```python
from build123d import *

# Parameters (mm, degrees)
SKETCH1_R           = 44.45
BOSS_EXTRUDE1_DEPTH = 55.88
SKETCH2_R           = 38.1
CUT_EXTRUDE1_DEPTH  = 22.098
CUT_EXTRUDE2_START  = -28.575
SKETCH3_R           = 38.1
CUT_EXTRUDE2_DEPTH  = 28.575
SKETCH4_R           = 1.27
CUT_EXTRUDE3_DEPTH  = 72.364056247
CUT_EXTRUDE4_DEPTH  = 5


with BuildPart() as part:
    # Sketch1 → Boss-Extrude1 (new body)
    with BuildSketch(Plane.XY):
        Circle(SKETCH1_R)
    extrude(amount=BOSS_EXTRUDE1_DEPTH)

    # Sketch2 → Cut-Extrude1 (cut)
    with BuildSketch(Plane.XY.offset(55.88)):
        Circle(SKETCH2_R)
    extrude(amount=-CUT_EXTRUDE1_DEPTH, mode=Mode.SUBTRACT)

    # Sketch3 → Cut-Extrude2 (cut)
    with BuildSketch(Plane(origin=(0, 0, 0), x_dir=(-1, 0, 0), z_dir=(0, 0, -1)).offset(CUT_EXTRUDE2_START)):
        with Locations(Location((0, 0, 0), (0, 0, 180))):
            Circle(SKETCH3_R)
    extrude(amount=CUT_EXTRUDE2_DEPTH, mode=Mode.SUBTRACT)

    # Sketch4 → Cut-Extrude3 (cut, through all)
    with BuildSketch(Plane.XY.offset(33.782)):
        Circle(SKETCH4_R)
    extrude(amount=-CUT_EXTRUDE3_DEPTH, mode=Mode.SUBTRACT)

    # Sketch5 → Cut-Extrude4 (cut)
    with BuildSketch(Plane.XY.offset(33.782)):
        Polygon((0, 8.082903769), (-7, 4.041451884), (-7, -4.041451884), (0, -8.082903769), (7, -4.041451884), (7, 4.041451884), align=None)
    extrude(amount=-CUT_EXTRUDE4_DEPTH, mode=Mode.SUBTRACT)


solid = part.part
```
Model file for the job. Use its own axes, mm. A direction names the side the tool comes from. Give positions to 0.01 mm unless a question says otherwise; leave off trailing zeros. Loops run counter-clockwise (first coordinate to the right, second up) from the corner with the lowest first, then second, coordinate; pieces in that order, holes last. Notation, with made-up numbers: (17, 16.25) -> (68, 16.25) arc R10 cw to (68, 22.25) -> close; hole circle Ø1 at (25, -17.75). An arc over 180 degrees is marked (long way). Use CSV: the item, a comma, the result in double quotes. Start each with the question number.
1) Mould opens along X. For faces 4 (the flat face through (33, 20, 0)), 5 (the cylindrical face through (42.397, 13.352, 27.549)), 6 (the flat face through (3.549, 6.034, 31.317)) say: released by +X, released by -X, zero draft, split by the parting line, or undercut.
2) Wall check: line 1 (Y direction, x = 0, z = 28); line 2 (Z direction, x = 22.5, y = -13.5) (3 decimals); line 3 (X direction, y = -14, z = 46.5). Give the ranges that are in metal, low to high.
3) Slice it at C-C on x = -23.5. Give the cut face in (y, z) (3 decimals).
4) Flat gauge pins, fed straight in: pin 1 Ø1 at (y, z) = (23.5, 19.5) entering from -X; pin 2 Ø4 at (x, y) = (-2.5, -1) entering from +Z; pin 3 Ø4 at (x, y) = (-15, -28) entering from -Z (3 decimals). Where does each tip first touch, or does it go through?
5) Slice it at B-B on z = 31. Give the cut face in (x, y).
6) Tool access for faces 1 (the flat face through (8, -1, 28.575)), 2 (the flat face through (33, 20, 55.88)), 3 (the flat face through (-3.549, -6.034, 31.317)): list every direction of +Z, -Z, +X, -X, +Y, -Y with a clear straight run to the whole face (end or side of a thin tool).
7) Slice it at D-D on y = -16. Give the cut face in (x, z) (1 decimal), plus the area to 3 significant figures.
8) Slice it at A-A on y = 0. Give the cut face in (x, z) (3 decimals), plus the area to 3 significant figures.
Computed values:
1,face 4,"zero draft"
1,face 5,"split by the parting line"
1,face 6,"undercut"
2,line 1,"y = -44.45 to -38.1, 38.1 to 44.45"
2,line 2,"z = 28.575 to 33.782"
2,line 3,"x = -42.19 to -35.43, 35.43 to 42.19"
3,outline,"(-37.73, 0) -> (-29.989, 0) -> (-29.989, 28.575) -> (29.989, 28.575) -> (29.989, 0) -> (37.73, 0) -> (37.73, 55.88) -> (29.989, 55.88) -> (29.989, 33.782) -> (-29.989, 33.782) -> (-29.989, 55.88) -> (-37.73, 55.88) -> close"
4,pin 1,"stops at x = -38.04"
4,pin 2,"stops at z = 28.78"
4,pin 3,"stops at z = 28.575"
5,outline,"circle Ø88.9 at (0, 0); hole (-7, -4.04) -> (0, -8.08) -> (7, -4.04) -> (7, 4.04) -> (0, 8.08) -> (-7, 4.04) -> close"
6,face 1,"-Z"
6,face 2,"+Z, +X, -X, +Y, -Y"
6,face 3,"+Z"
7,outline,"(-41.5, 0) -> (-34.6, 0) -> (-34.6, 28.6) -> (34.6, 28.6) -> (34.6, 0) -> (41.5, 0) -> (41.5, 55.9) -> (34.6, 55.9) -> (34.6, 33.8) -> (-34.6, 33.8) -> (-34.6, 55.9) -> (-41.5, 55.9) -> close"
7,area,"1,130 mm^2"
8,outline,"(-44.45, 0) -> (-38.1, 0) -> (-38.1, 28.575) -> (-1.27, 28.575) -> (-1.27, 28.782) -> (-7, 28.782) -> (-7, 33.782) -> (-38.1, 33.782) -> (-38.1, 55.88) -> (-44.45, 55.88) -> close; (1.27, 28.575) -> (38.1, 28.575) -> (38.1, 0) -> (44.45, 0) -> (44.45, 55.88) -> (38.1, 55.88) -> (38.1, 33.782) -> (7, 33.782) -> (7, 28.782) -> (1.27, 28.782) -> close"
8,area,"1,040 mm^2"
